Design review of the part built by this model. Coordinates are the model's own, in mm. A direction names the side the tool comes from. Give positions to 0.01 mm unless a question says otherwise; leave off trailing zeros. Write each loop counter-clockwise with the first axis right and the second up, starting at its lowest first coordinate (ties: lowest second). Pieces come first, ordered by that corner, then holes. Notation, with made-up numbers: (-23.75, -27.75) -> (21.25, -27.75) arc R28 ccw to (21.25, 4.25) -> close; hole circle Ø2 at (51.25, -4). An arc over 180 degrees is marked (long way). Answer as a JSON object with one key per item and string values.
```python
from build123d import *

# Parameters (mm, degrees)
SKETCH1_W           = 15
SKETCH1_H           = 15
SKETCH1_W_2         = 10.56
SKETCH1_H_2         = 5
BOSS_EXTRUDE1_DEPTH = 1.6
SKETCH1_3_W         = 10.56
SKETCH1_3_H         = 5
BOSS_EXTRUDE2_DEPTH = 2
BOSS_EXTRUDE3_DEPTH = 8.6


with BuildPart() as part:
    # Sketch1 → Boss-Extrude1 (new body)
    # profile 1 of 3: a face of its own
    with BuildSketch(Plane(origin=(0, 0, 0), x_dir=(1, 0, 0), z_dir=(0, 1, 0))):
        with Locations((0, 3)):
            Rectangle(SKETCH1_W, SKETCH1_H)
        Rectangle(SKETCH1_W_2, SKETCH1_H_2, mode=Mode.SUBTRACT)
    # profile 2 of 3: a face of its own
    with BuildSketch(Plane(origin=(0, 0, 0), x_dir=(1, 0, 0), z_dir=(0, 1, 0))):
        Rectangle(SKETCH1_W_2, SKETCH1_H_2)
    # profile 3 of 3: a face of its own
    with BuildSketch(Plane(origin=(0, 0, 0), x_dir=(1, 0, 0), z_dir=(0, 1, 0))):
        Polygon((-50, 10.5), (-7.5, 10.5), (7.5, 10.5), (50, 10.5), (50, 25.5), (-50, 25.5), align=None)
        Polygon((-42.569302237, 23.1), (-41.1, 21.630697763), (-41.1, 12.9), (-46.9, 12.9), (-46.9, 21.630697763), (-45.430697763, 23.1), align=None, mode=Mode.SUBTRACT)
        Polygon((-20.569302237, 23.1), (-19.1, 21.630697763), (-19.1, 12.9), (-24.9, 12.9), (-24.9, 21.630697763), (-23.430697763, 23.1), align=None, mode=Mode.SUBTRACT)
        Polygon((2.9, 12.9), (-2.9, 12.9), (-2.9, 21.630697763), (-1.430697763, 23.1), (1.430697763, 23.1), (2.9, 21.630697763), align=None, mode=Mode.SUBTRACT)
        Polygon((23.430697763, 23.1), (24.9, 21.630697763), (24.9, 12.9), (19.1, 12.9), (19.1, 21.630697763), (20.569302237, 23.1), align=None, mode=Mode.SUBTRACT)
        Polygon((45.430697763, 23.1), (46.9, 21.630697763), (46.9, 12.9), (41.1, 12.9), (41.1, 21.630697763), (42.569302237, 23.1), align=None, mode=Mode.SUBTRACT)
    extrude(amount=BOSS_EXTRUDE1_DEPTH)

    # Sketch1_3 → Boss-Extrude2 (add)
    with BuildSketch(Plane(origin=(0, 0, 0), x_dir=(1, 0, 0), z_dir=(0, 1, 0))):
        Rectangle(SKETCH1_3_W, SKETCH1_3_H)
    extrude(amount=-BOSS_EXTRUDE2_DEPTH)

    # Sketch1_4 → Boss-Extrude3 (add)
    with BuildSketch(Plane(origin=(0, 0, 0), x_dir=(1, 0, 0), z_dir=(0, 1, 0))):
        Polygon((23.430697763, 23.1), (24.9, 21.630697763), (24.9, 12.9), (19.1, 12.9), (19.1, 21.630697763), (20.569302237, 23.1), align=None)
        Polygon((45.430697763, 23.1), (46.9, 21.630697763), (46.9, 12.9), (41.1, 12.9), (41.1, 21.630697763), (42.569302237, 23.1), align=None)
        Polygon((2.9, 21.630697763), (2.9, 12.9), (-2.9, 12.9), (-2.9, 21.630697763), (-1.430697763, 23.1), (1.430697763, 23.1), align=None)
        Polygon((-20.569302237, 23.1), (-19.1, 21.630697763), (-19.1, 12.9), (-24.9, 12.9), (-24.9, 21.630697763), (-23.430697763, 23.1), align=None)
        Polygon((-42.569302237, 23.1), (-41.1, 21.630697763), (-41.1, 12.9), (-46.9, 12.9), (-46.9, 21.630697763), (-45.430697763, 23.1), align=None)
    extrude(amount=BOSS_EXTRUDE3_DEPTH)

    # Sketch3 → Revolve2 (revolve)
    with BuildSketch(Plane(origin=(0, 0, 0), x_dir=(0, 0, -1), z_dir=(1, 0, 0))):
        with BuildLine():
            add(Edge.make_bspline(
                [(-1.5, 1.6), (-1.5, 8.223178145), (1, 11.999705618), (3.5, 12.1)],
                knots=[0, 0, 0, 0, 0.5, 0.5, 0.5, 0.5], degree=3))
            Line((-1.5, 1.6), (3.5, 1.6))
            Line((3.5, 1.6), (3.5, 12.1))
        make_face()
    revolve(axis=Axis((0, 12.1, -3.5), (0, -1, 0)))


solid = part.part
```
(1) We need section C-C, the plane y = 6.25. Give the number of separate pieces and of enclosed holes in the cut face, then the cut area to 3 significant figures.
Here are the results:
{"separate pieces": "6", "enclosed holes": "0", "area": "349 mm²"}
(2) The part is to be moulded in two halves that separate along X. For faces 5 (the flat face through (46.9, 5, -17)), 6 (the flat face through (22, 5, -23.1)), 7 (the flat face through (-24.9, 5, -17)), say which applies: +X half, -X half, draft (parallel to the pull), parting line (faces both ways), or undercut.
Here are the results:
{"face 5": "+X half", "face 6": "draft", "face 7": "undercut"}
(3) For faces 1 (the flat face through (-29, 1, -10.5)), 2 (the flat face through (44, 5, -23.1)), 3 (the flat face through (22, 5, -12.9)), 4 (the flat face through (-46.9, 5, -17)), list the 3-axis set-ups (+Z, -Z, +X, -X, +Y, -Y) from which the entire face can be reached by the end or side of a thin tool; tool diameter is ignored.
Here are the results:
{"face 1": "+Z, -X, +Y, -Y", "face 2": "-Z, +X, -X, +Y", "face 3": "+Z, +X, -X, +Y", "face 4": "+Z, -Z, -X, +Y"}
(4) Clearance check with flat-ended pins moving along their axes: pin 1 (1.7 mm diameter, centred on x = 0, y = 4, fed in from +Z); pin 2 (3 mm diameter, centred on x = -43.5, y = 6, fed in from -Z); pin 3 (2 mm diameter, centred on y = 3.5, z = -18, fed in from +X); pin 4 (15 mm diameter, centred on x = 1.5, z = -5, fed in from -Y). State where each tip first meets the part, or that it passes through.
Here are the results:
{"pin 1": "stops at z = 1.45", "pin 2": "stops at z = -23.1", "pin 3": "stops at x = 46.9", "pin 4": "stops at y = -2"}
(5) For line 1 along X through (y, z) = (4.75, -16.5); line 2 along Y through (x, z) = (-38.5, -14.75); line 3 along Z through (x, y) = (-20, 0.5), list the stretches that pass through material, from the lowest coordinate up.
Here are the results:
{"line 1": "x = -46.9 to -41.1, -24.9 to -19.1, -2.9 to 2.9, 19.1 to 24.9, 41.1 to 46.9", "line 2": "y = 0 to 1.6", "line 3": "z = -25.5 to -10.5"}
(6) We need section A-A, the plane x = 22.5. State the section outline as (y, z) points.
Here are the results:
{"outline": "(0, -25.5) -> (1.6, -25.5) -> (1.6, -23.1) -> (8.6, -23.1) -> (8.6, -12.9) -> (1.6, -12.9) -> (1.6, -10.5) -> (0, -10.5) -> close"}
(7) We need section B-B, the plane z = -20.25. State the section outline as (x, y) points, then the cut area to 3 significant figures.
Here are the results:
{"outline": "(-50, 0) -> (50, 0) -> (50, 1.6) -> (46.9, 1.6) -> (46.9, 8.6) -> (41.1, 8.6) -> (41.1, 1.6) -> (24.9, 1.6) -> (24.9, 8.6) -> (19.1, 8.6) -> (19.1, 1.6) -> (2.9, 1.6) -> (2.9, 8.6) -> (-2.9, 8.6) -> (-2.9, 1.6) -> (-19.1, 1.6) -> (-19.1, 8.6) -> (-24.9, 8.6) -> (-24.9, 1.6) -> (-41.1, 1.6) -> (-41.1, 8.6) -> (-46.9, 8.6) -> (-46.9, 1.6) -> (-50, 1.6) -> close", "area": "363 mm²"}
